Verification items for the finished model (mm, model axes). Face numbers are marked on the shaded views. Give positions to 0.01 mm unless a question says otherwise; leave off trailing zeros. Order: outer loops, then holes, each group sorted by start corner. A loop starts at its lowest first (then second) coordinate and runs counter-clockwise, first axis right, second up. Notation, with made-up numbers: (68, -20) -> (105, -20) arc R9 cw to (105, -6) -> close; hole circle Ø7 at (-17.5, 35.5). An arc over 180 degrees is marked (long way). Return JSON: item names as keys, results as strings. Group by question number.
(1) Cross-section at C-C on x = -30. Enter the section's corners in (y, z).
(2) Thickness scan on line 1 along Z through (x, y) = (-87, 5.75); line 2 along Z through (x, y) = (30, 4); line 3 along Z through (x, y) = (-83.5, 4.25). Record the ranges inside material, lowest first.
(3) Depth check by flat-ended pin: pin 1 Ø3.5 at (y, z) = (7, -1) entering from +X; pin 2 Ø4.5 at (x, z) = (30, 40) entering from +Y; pin 3 Ø5 at (x, z) = (-17.5, 0) entering from +Y. Enter the tip coordinate at first touch or a pass-through.
(4) Cross-section at A-A on x = 87. Enter the section's corners in (y, z), then the cut area to 3 significant figures.
(5) Cross-section at D-D on y = 3.25. State how many separate pieces and enclosed holes the cut face has, then the cut area to 3 significant figures.
(6) Release check for a two-part mould opening along X. For the marked faces 1 and 2 record: pulls with the +X half, pulls with the -X half, needs draft (parallel to the pull), parting line crosses it, or undercut.
(7) Cross-section at B-B on z = 7.5. Enter the section's corners in (x, y), then the cut area to 3 significant figures.
from build123d import *

# Parameters (mm, degrees)
SKETCH1_W               = 120
SKETCH1_H               = 100
BOSS_EXTRUDE1_DEPTH     = 5
SKETCH2_W               = 120
SKETCH2_H               = 100
SKETCH2_W_2             = 85
SKETCH2_H_2             = 57
BOSS_EXTRUDE2_DEPTH     = 5
SKETCH3_W               = 35
SKETCH3_H               = 17
BOSS_EXTRUDE3_DEPTH     = 10
CUT_EXTRUDE1_DEPTH      = 108.819293264
CUT_EXTRUDE1_DEPTH_BACK = 108.819293264
SKETCH4_R               = 2.95
FILLET1_R               = 2
CUT_EXTRUDE2_DEPTH      = 108.819293264
CUT_EXTRUDE2_DEPTH_BACK = 108.819293264
SKETCH5_R               = 3.75


with BuildPart() as part:
    # Sketch1 → Boss-Extrude1 (new body)
    with BuildSketch(Plane(origin=(0, 0, 0), x_dir=(1, 0, 0), z_dir=(0, 1, 0))):
        Rectangle(SKETCH1_W, SKETCH1_H)
    extrude(amount=BOSS_EXTRUDE1_DEPTH)

    # Sketch2 → Boss-Extrude2 (add)
    with BuildSketch(Plane(origin=(0, 5, 0), x_dir=(1, 0, 0), z_dir=(0, 1, 0))):
        Rectangle(SKETCH2_W, SKETCH2_H)
        Rectangle(SKETCH2_W_2, SKETCH2_H_2, mode=Mode.SUBTRACT)
    extrude(amount=BOSS_EXTRUDE2_DEPTH)

    # Sketch3 → Boss-Extrude3 (add)
    with BuildSketch(Plane.XZ):
        with Locations((77.5, 41.5)):
            Rectangle(SKETCH3_W, SKETCH3_H)
        with Locations((77.5, -41.5)):
            Rectangle(SKETCH3_W, SKETCH3_H)
        with Locations((-77.5, -41.5)):
            Rectangle(SKETCH3_W, SKETCH3_H)
        with Locations((-77.5, 41.5)):
            Rectangle(SKETCH3_W, SKETCH3_H)
    extrude(amount=-BOSS_EXTRUDE3_DEPTH)

    # Sketch4 → Cut-Extrude1 (cut, two sides: drawn at the far end of the back side and taken through both)
    with BuildSketch(Plane.XZ.offset(-CUT_EXTRUDE1_DEPTH_BACK)):
        with Locations(Location((70, 37.5, 0), (0, 0, 270))):
            Circle(SKETCH4_R)
        with Locations(Location((87, 37.5, 0), (0, 0, 270))):
            Circle(SKETCH4_R)
        with Locations(Location((70, -37.5, 0), (0, 0, 270))):
            Circle(SKETCH4_R)
        with Locations(Location((87, -37.5, 0), (0, 0, 270))):
            Circle(SKETCH4_R)
        with Locations(Location((-87, -37.5, 0), (0, 0, 270))):
            Circle(SKETCH4_R)
        with Locations(Location((-70, -37.5, 0), (0, 0, 270))):
            Circle(SKETCH4_R)
        with Locations(Location((-87, 37.5, 0), (0, 0, 270))):
            Circle(SKETCH4_R)
        with Locations(Location((-70, 37.5, 0), (0, 0, 270))):
            Circle(SKETCH4_R)
    extrude(amount=CUT_EXTRUDE1_DEPTH + CUT_EXTRUDE1_DEPTH_BACK, mode=Mode.SUBTRACT)

    # Fillet1
    fillet1_edges = [part.edges().sort_by_distance(p)[0] for p in [
        (42.5, 10, 0),
        (0, 10, -28.5),
        (-42.5, 10, 0),
        (0, 10, 28.5),
        (95, 5, 50),
        (95, 5, 33),
        (95, 5, -33),
        (95, 5, -50),
        (-95, 5, -50),
        (-95, 5, -33),
        (-95, 5, 50),
        (-95, 5, 33),
    ]]
    fillet(fillet1_edges, radius=FILLET1_R)

    # Sketch5 → Cut-Extrude2 (cut, two sides: drawn at the far end of the back side and taken through both)
    with BuildSketch(Plane(origin=(0, 10, 0), x_dir=(1, 0, 0), z_dir=(0, 1, 0)).offset(-CUT_EXTRUDE2_DEPTH_BACK)):
        with Locations(Location((-30, 40, 0), (0, 0, 270))):
            Circle(SKETCH5_R)
        with Locations(Location((30, 40, 0), (0, 0, 270))):
            Circle(SKETCH5_R)
        with Locations(Location((-30, -40, 0), (0, 0, 270))):
            Circle(SKETCH5_R)
        with Locations(Location((30, -40, 0), (0, 0, 270))):
            Circle(SKETCH5_R)
    extrude(amount=CUT_EXTRUDE2_DEPTH + CUT_EXTRUDE2_DEPTH_BACK, mode=Mode.SUBTRACT)


solid = part.part
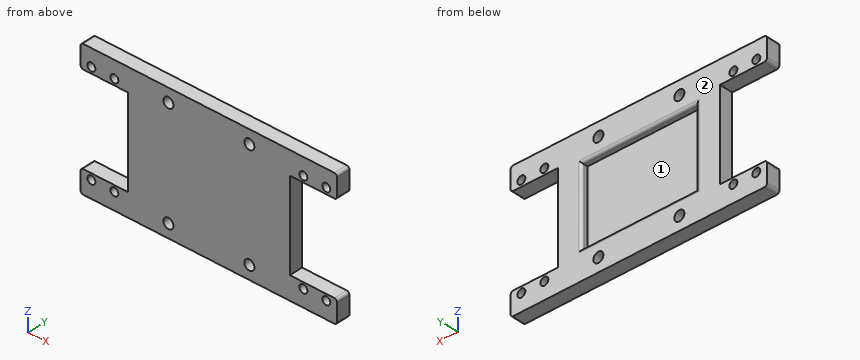
Verdict:
{
 "1": {"outline": "(0, -50) -> (10, -50) -> (10, -43.75) -> (0, -43.75) -> close; (0, -36.25) -> (10, -36.25) -> (10, -30.5) arc R2 ccw to (8, -28.5) -> (5, -28.5) -> (5, 28.5) -> (8, 28.5) arc R2 ccw to (10, 30.5) -> (10, 36.25) -> (0, 36.25) -> close; (0, 43.75) -> (10, 43.75) -> (10, 50) -> (0, 50) -> close"},
 "2": {"line 1": "-50 to -40.45, -34.55 to -33, 33 to 34.55, 40.45 to 50", "line 2": "-50 to -43.75, -36.25 to 36.25, 43.75 to 50", "line 3": "-50 to -33, 33 to 50"},
 "3": {"pin 1": "x = 60", "pin 2": "through", "pin 3": "y = 5"},
 "4": {"outline": "(0, -50) -> (10, -50) -> (10, -40.45) -> (0, -40.45) -> close; (0, -34.55) -> (10, -34.55) -> (10, -33) -> (0, -33) -> close; (0, 33) -> (10, 33) -> (10, 34.55) -> (0, 34.55) -> close; (0, 40.45) -> (10, 40.45) -> (10, 50) -> (0, 50) -> close", "area": "222 mm²"},
 "5": {"separate pieces": "1", "enclosed holes": "12", "area": "14,000 mm²"},
 "6": {"face 1": "undercut", "face 2": "needs draft"},
 "7": {"outline": "(-60, 0) -> (60, 0) -> (60, 10) -> (44.5, 10) arc R2 ccw to (42.5, 8) -> (42.5, 5) -> (-42.5, 5) -> (-42.5, 8) arc R2 ccw to (-44.5, 10) -> (-60, 10) -> close", "area": "773 mm²"}
}
